Geometry check sheet. Reference: the model listing, model coordinates, mm. Round coordinates to 2 decimals unless told otherwise and drop trailing zeros. Order: outer loops, then holes, each group sorted by start corner. A loop starts at its lowest first (then second) coordinate and runs counter-clockwise, first axis right, second up. Notation, with made-up numbers: (59, 33) -> (69, 33) arc R31 ccw to (69, 65) -> close; hole circle Ø4 at (41, 40.5). An arc over 180 degrees is marked (long way). Use a Markdown table: item, result. Add a question column.
Item 1: Gauge pin test, flat ends, axial feed: pin 1 Ø8 at (y, z) = (4, -15) entering from +X; pin 2 Ø8 at (x, y) = (1.5, 1.5) entering from -Z; pin 3 Ø2 at (y, z) = (2.5, -10) entering from +X; pin 4 Ø4 at (y, z) = (-3, -29.5) entering from -X. Record the tip position at first contact, or that the pin passes through.
Item 2: Sectioned sample at B-B, the plane z = 20. Record the cut outline in (x, y), and give its area (3 significant figures).
Item 3: Sectioned sample at D-D, the plane z = -33. Record the cut outline in (x, y), and give its area (3 significant figures).
Item 4: Material ranges on probe 1 along Z at (x, y) = (-5, 3.5) (3 decimals); probe 2 along X at (y, z) = (-1.75, -25) (3 decimals); probe 3 along X at (y, z) = (-5.25, 14.5), recorded low to high. Write a range as [from, to].
Item 5: Sectioned sample at C-C, the plane x = 25. Record the cut outline in (y, z).
Item 6: Sectioned sample at A-A, the plane y = -2. Record the cut outline in (x, z), and give its area (3 significant figures).
from build123d import *

# Parameters (mm, degrees)
F0_R     = 8
F1_DEPTH = 7.5


# Not quite as in the source:
# - the program builds the solid bodies; features that only make, move or delete a surface that nothing else refers to are left out


with BuildPart() as f1:
    # F0 (on Front) → F1 (new body, symmetric)
    with BuildSketch(Plane.XZ):
        with BuildLine():
            ThreePointArc((0, -40), (28.2842712475, -28.2842712475), (40, 0))
            ThreePointArc((40, 0), (28.2842712475, 28.2842712475), (0, 40))
            ThreePointArc((0, 40), (-20, 20), (0, 0))
            ThreePointArc((0, 0), (20, -20), (0, -40))
        make_face()
        with Locations((0, 20)):
            Circle(F0_R, mode=Mode.SUBTRACT)
        with BuildLine():
            ThreePointArc((0, 0), (-20, 20), (0, 40))
            ThreePointArc((0, 40), (-40, 0), (0, -40))
            ThreePointArc((0, -40), (20, -20), (0, 0))
        make_face()
        with Locations((0, -20)):
            Circle(F0_R, mode=Mode.SUBTRACT)
    extrude(amount=F1_DEPTH, both=True)


solid = f1.part
Found:
| question | item | result |
|---|---|---|
| 1 | pin 1 | stops at x = 38.46 |
| 1 | pin 2 | stops at z = -40 |
| 1 | pin 3 | stops at x = 38.97 |
| 1 | pin 4 | stops at x = -29.05 |
| 2 | outline | (-34.64, -7.5) -> (-8, -7.5) -> (-8, 7.5) -> (-34.64, 7.5) -> close; (8, -7.5) -> (34.64, -7.5) -> (34.64, 7.5) -> (8, 7.5) -> close |
| 2 | area | 799 mm2 |
| 3 | outline | (-22.61, -7.5) -> (22.61, -7.5) -> (22.61, 7.5) -> (-22.61, 7.5) -> close |
| 3 | area | 678 mm2 |
| 4 | probe 1 | z = [-39.686, -26.245], [-13.755, 13.755], [26.245, 39.686] |
| 4 | probe 2 | x = [-31.225, -6.245], [6.245, 31.225] |
| 4 | probe 3 | x = [-37.28, -5.81], [5.81, 37.28] |
| 5 | outline | (-7.5, -31.22) -> (7.5, -31.22) -> (7.5, 31.22) -> (-7.5, 31.22) -> close |
| 6 | outline | circle Ø80 at (0, 0); hole circle Ø16 at (0, -20); hole circle Ø16 at (0, 20) |
| 6 | area | 4,620 mm2 |
